Autodesk Inventor part; units mm, degrees
ref_plane "1_XY" through (0, 5.7912, 0) normal (0, 1, 0) x (1, 0, 0)
ref_plane "1_YZ" through (0, 5.7912, 0) normal (1, 0, 0) x (0, 0, -1)
ref_plane "1_ZX" through (0, 5.7912, 0) normal (0, 0, -1) x (0, 1, 0)
sketch "Sketch_1" plane through (0, 0, 0) normal (0, 0, 1) x (1, 0, 0)
  line L0 (-3.9497, 0) -> (3.9497, 0)
  arc A0 (3.9497, 0) -> (3.6957, 0.254) centre (3.6957, 0) ccw
  line L1 (3.6957, 0.254) -> (-3.6957, 0.254)
  arc A1 (-3.6957, 0.254) -> (-3.9497, 0) centre (-3.6957, 0) ccw
extrude "Extrusion1" add sketch "Sketch_1" along normal mid plane 13.0048
sketch "Sketch_7" plane through (0, 0, 0) normal (0, 0, 1) x (1, 0, 0)
  line L0 (0, 0.127) -> (0, 7.62)
  line L1 (0, 7.62) -> (2.479, 7.62)
  line L2 (2.479, 7.62) -> (3.0988, 7.0002)
  line L3 (3.0988, 7.0002) -> (3.0988, 1.397)
  line L4 (3.0988, 1.397) -> (4.0005, 1.397)
  line L5 (4.0005, 1.397) -> (4.0005, 0.508)
  line L6 (4.0005, 0.508) -> (3.2537, 0.508)
  line L7 (3.2537, 0.508) -> (3.2537, 0.127)
  line L8 (3.2537, 0.127) -> (0, 0.127)
  line L9 (0, 0.127) -> (0, 7.62)
revolve "Revolution1" add sketch "Sketch_7" angle 360 about axis through (0, 0.127, 0) along (0, -1, 0)
sketch "Sketch_8" plane through (0, 0.254, 0) normal (0, 1, 0) x (1, 0, 0)
  line L0 (-0.3937, 2.4892) -> (0.3937, 2.4892)
  line L1 (0.3937, 2.4892) -> (0.3937, 10.4902)
  line L2 (0.3937, 10.4902) -> (-0.3937, 10.4902)
  line L3 (-0.3937, 10.4902) -> (-0.3937, 2.4892)
extrude "Extrusion2" cut sketch "Sketch_8" along normal blind 7.9629
sketch "Sketch4" plane through (-3.9497, 0, 6.5024) normal (0, -1, 0) x (1, 0, 0)
  point P0 (3.9497, -6.5024)
hole "Drilling 1" at (0, 0, 0) direction (0, 1, 0) diameter 4.3383 depth 7.874
sketch "Sketch_2" plane through (0, 0, 0) normal (0, 0, 1) x (1, 0, 0)
  line L0 (-3.9497, 0.254) -> (-3.9497, 0)
  line L1 (-3.9497, 0) -> (3.9497, 0)
  line L2 (3.9497, 0) -> (3.9497, 0.254)
  line L3 (3.9497, 0.254) -> (-3.9497, 0.254)
extrude "Extrusion3" cut sketch "Sketch_2" along normal mid plane 13.0048
ref_plane "1_XY" through (0, 5.7912, 0) normal (0, 1, 0) x (1, 0, 0)
ref_plane "1_YZ" through (0, 5.7912, 0) normal (1, 0, 0) x (0, 0, -1)
ref_plane "1_ZX" through (0, 5.7912, 0) normal (0, 0, -1) x (0, 1, 0)
ref_plane "2_XY" through (0, 4.3434, 0) normal (0, 1, 0) x (1, 0, 0)
ref_plane "2_YZ" through (0, 4.3434, 0) normal (1, 0, 0) x (0, 0, -1)
ref_plane "2_ZX" through (0, 4.3434, 0) normal (0, 0, -1) x (0, 1, 0)
ref_plane "3_XY" through (0, 2.8956, 0) normal (0, 1, 0) x (1, 0, 0)
ref_plane "3_YZ" through (0, 2.8956, 0) normal (1, 0, 0) x (0, 0, -1)
ref_plane "3_ZX" through (0, 2.8956, 0) normal (0, 0, -1) x (0, 1, 0)
ref_plane "4_XY" through (0, 1.8097, 0) normal (0, 1, 0) x (1, 0, 0)
ref_plane "4_YZ" through (0, 1.8097, 0) normal (1, 0, 0) x (0, 0, -1)
ref_plane "4_ZX" through (0, 1.8097, 0) normal (0, 0, -1) x (0, 1, 0)
ref_plane "to_base_XY" through (0, 0, 0) normal (0, 1, 0) x (1, 0, 0)
ref_plane "to_base_YZ" through (0, 0, 0) normal (1, 0, 0) x (0, 0, -1)
ref_plane "to_base_ZX" through (0, 0, 0) normal (0, 0, -1) x (0, 1, 0)
properties part number "M20ANG1A2M201BR-bushing"
The listing builds one solid part. Answer for the finished solid, in the listing's coordinates (mm). A direction names the side the tool comes from. Coordinates: 2 decimals unless noted, no trailing zeros. Write each loop counter-clockwise with the first axis right and the second up, starting at its lowest first coordinate (ties: lowest second). Pieces come first, ordered by that corner, then holes. Notation, with made-up numbers: (20.5, 36) - (37.5, 36) arc R3 ccw to (37.5, 41) - close; hole circle Ø3 at (3, 46.5). An arc over 180 degrees is marked (long way). One line per item, written item: value.
1) A tool of negligible diameter and unlimited length cuts with its end or side. For faces 1 (the flat face through (-0.394, 3.1, -2.9)), 2 (the cylindrical face through (0.131, 4.159, 3.096)), from which of +Z, -Z, +X, -X, +Y, -Y can it reach the whole face along a straight path? Write none if from no direction.
Geometry check:
face 1: -Z, +Y, -Y
face 2: +Y
2) Each of these flat-tipped pins is pushed along its axis until it touches: pin 1 Ø1 at (x, y) = (2.5, 5) entering from -Z; pin 2 Ø4 at (x, y) = (-2, 2) entering from +Z; pin 3 Ø2.5 at (x, z) = (0, 0) entering from +Y; pin 4 Ø4 at (y, z) = (5, 3) entering from +X. Where does it stop, or does it pass through?
Geometry check:
pin 1: stops at z = -2.37
pin 2: stops at z = 4
pin 3: passes through
pin 4: stops at x = 2.93
3) Find section B-B (z = 0). Give the vertices of the cut face in (x, y).
Geometry check:
outline: (-4, 0.51) - (-3.25, 0.51) - (-3.25, 0.25) - (-2.17, 0.25) - (-2.17, 7.62) - (-2.48, 7.62) - (-3.1, 7) - (-3.1, 1.4) - (-4, 1.4) - close; (2.17, 0.25) - (3.25, 0.25) - (3.25, 0.51) - (4, 0.51) - (4, 1.4) - (3.1, 1.4) - (3.1, 7) - (2.48, 7.62) - (2.17, 7.62) - close
4) Find section C-C (y = 6). Give the vertices of the cut face in (x, z).
Geometry check:
outline: (-0.39, -3.07) - (-0.39, -2.49) - (0.39, -2.49) - (0.39, -3.07) arc R3.1 ccw (long way) to start; hole circle Ø4.34 at (0, 0)
5) For a pull along Z with two mould halves and no side action, classify faces 3 (the cylindrical face through (0, 1, 4)), 4 (the cylindrical face through (-0.65, 3.99, -2.07)), 5 (the flat face through (-2, 0.508, -3)) as pulls with the +Z half, pulls with the -Z half, needs draft (parallel to the pull), parting line crosses it, or undercut.
Geometry check:
face 3: parting line crosses it
face 4: undercut
face 5: needs draft
6) Find section D-D (z = -3.5). Give the vertices of the cut face in (x, y), and give its area (3 significant figures).
Geometry check:
outline: (-1.94, 0.51) - (-0.39, 0.51) - (-0.39, 1.4) - (-1.94, 1.4) - close; (0.39, 0.51) - (1.94, 0.51) - (1.94, 1.4) - (0.39, 1.4) - close
area: 2.74 mm2
7) Consider line 1 along Z through (x, y) = (0, 4.5); line 2 along X through (y, z) = (2, 0); line 3 along X through (y, z) = (1.5, -1). Determine where each line is inside the solid, lowest interval first. Write a range as from..to.
Geometry check:
line 1: z = -2.49..-2.17, 2.17..3.1
line 2: x = -3.1..-2.17, 2.17..3.1
line 3: x = -2.93..-1.92, 1.92..2.93
